Geometry check sheet. Reference: the model listing, model coordinates, mm. Face numbers are marked on the shaded views. A direction names the side the tool comes from. Round coordinates to 2 decimals unless told otherwise and drop trailing zeros. Order: outer loops, then holes, each group sorted by start corner. A loop starts at its lowest first (then second) coordinate and runs counter-clockwise, first axis right, second up.
(1) Cross-section at B-B on z = -37. Enter the section's corners in (x, y).
(2) Set-up check for the marked faces 4, 5 and 6: record each of +Z, -Z, +X, -X, +Y, -Y from which the full face is reachable in a straight line by a thin tool's end or side.
(3) Thickness scan on L1, parallel to X at y = -14.65, z = -37; L2, parallel to Z at x = 47.5, y = -14.25; L3, parallel to Z at x = 12, y = -5. Record the ranges inside material, lowest first.
(4) Cross-section at C-C on y = -2. Enter the section's corners in (x, z).
(5) Draft check along Z on the marked faces 1, 2 and 3. Enter one of: pulls with the +Z half, pulls with the -Z half, needs draft (parallel to the pull), parting line crosses it, or undercut.
(6) Gauge pin test, flat end, axial feed: P1, Ø4.5, axis at x = 25, z = -25, coming from the -Y side. Record the tip position at first contact, or that the pin passes through.
(7) Cross-section at D-D on z = -47. Enter the section's corners in (x, y), and give its area (3 significant figures).
(8) Cross-section at A-A on x = 20. Enter the section's corners in (y, z).
from build123d import *

# Parameters (mm, degrees)
SKETCH_R        = 3.2
SKETCH_R_2      = 1.98
SKETCH_R_3      = 12.5
PAD_DEPTH       = 18.5
SKETCH001_R     = 4.7
POCKET_DEPTH    = 6
SKETCH002_R     = 16
POCKET001_DEPTH = 13.1
SKETCH003_R     = 6
POCKET002_DEPTH = 55


with BuildPart() as part:
    # Sketch → Pad (new body)
    with BuildSketch(Plane.XZ):
        Polygon((0, 0), (0, -57), (50.5, -57), (64.5, -43), (64.5, -18.5), (46, 0), align=None)
        with Locations((10, -7)):
            Circle(SKETCH_R, mode=Mode.SUBTRACT)
        with Locations((20, -47)):
            Circle(SKETCH_R, mode=Mode.SUBTRACT)
        with Locations((25, -25)):
            Circle(SKETCH_R_2, mode=Mode.SUBTRACT)
        with Locations((45, -37)):
            Circle(SKETCH_R_3, mode=Mode.SUBTRACT)
    extrude(amount=PAD_DEPTH)

    # Sketch001 → Pocket (cut)
    with BuildSketch(Plane.XZ.offset(18.5)):
        with Locations((10, -7)):
            Circle(SKETCH001_R)
        with Locations((20, -47)):
            Circle(SKETCH001_R)
    extrude(amount=-POCKET_DEPTH, mode=Mode.SUBTRACT)

    # Sketch002 → Pocket001 (cut)
    with BuildSketch(Plane(origin=(0, 0, 0), x_dir=(1, 0, 0), z_dir=(0, 1, 0))):
        with Locations((45, 37)):
            Circle(SKETCH002_R)
    extrude(amount=-POCKET001_DEPTH, mode=Mode.SUBTRACT)

    # Sketch003 → Pocket002 (cut)
    with BuildSketch(Plane(origin=(0, 0, 0), x_dir=(0, 0, -1), z_dir=(-1, 0, 0))):
        with Locations((18.5, 9.25)):
            Circle(SKETCH003_R)
    extrude(amount=-POCKET002_DEPTH, mode=Mode.SUBTRACT)


solid = part.part
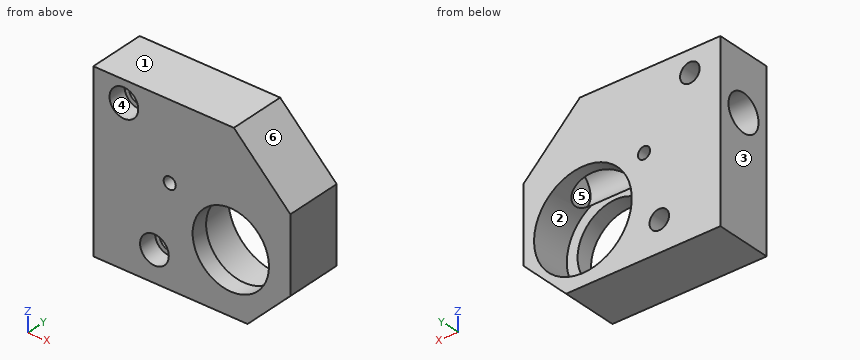
Found:
1. outline: (0, -18.5) - (32.5, -18.5) - (32.5, -13.1) - (29, -13.1) - (29, 0) - (0, 0) - close; (57.5, -18.5) - (64.5, -18.5) - (64.5, 0) - (61, 0) - (61, -13.1) - (57.5, -13.1) - close
2. face 4: -Y
2. face 5: -X
2. face 6: +Z, +X, +Y, -Y
3. L1: x = 0 to 32.5, 57.5 to 64.5
3. L2: z = -57 to -49.25, -24.75 to -21.82, -15.18 to -1.5
3. L3: z = -57 to -22.74, -14.26 to -9.5, -4.5 to 0
4. outline: (0, -57) - (50.5, -57) - (64.5, -43) - (64.5, -18.5) - (46, 0) - (0, 0) - close; hole circle Ø6.4 at (10, -7); hole circle Ø6.4 at (20, -47); hole circle Ø3.96 at (25, -25); hole circle Ø32 at (45, -37)
5. face 1: pulls with the +Z half
5. face 2: undercut
5. face 3: needs draft
6. P1: stops at y = -18.5
7. outline: (0, -18.5) - (15.3, -18.5) - (15.3, -12.5) - (16.8, -12.5) - (16.8, 0) - (0, 0) - close; (23.2, -12.5) - (24.7, -12.5) - (24.7, -18.5) - (37.5, -18.5) - (37.5, -13.1) - (32.51, -13.1) - (32.51, 0) - (23.2, 0) - close; (52.5, -18.5) - (60.5, -18.5) - (60.5, 0) - (57.49, 0) - (57.49, -13.1) - (52.5, -13.1) - close
7. area: 575 mm2
8. outline: (-18.5, -57) - (0, -57) - (0, -50.2) - (-12.5, -50.2) - (-12.5, -51.7) - (-18.5, -51.7) - close; (-18.5, -42.3) - (-12.5, -42.3) - (-12.5, -43.8) - (0, -43.8) - (0, 0) - (-18.5, 0) - close; hole circle Ø12 at (-9.25, -18.5)
